The listing builds one solid part. Answer for the finished solid, in the listing's coordinates (mm). Face numbers are marked on the shaded views. Round coordinates to 2 decimals unless told otherwise and drop trailing zeros. Order: outer loops, then holes, each group sorted by start corner. A loop starts at its lowest first (then second) coordinate and runs counter-clockwise, first axis right, second up. Notation, with made-up numbers: M 64,24 L 122,24 A15 ccw 122,28 Z; hole C 48,89 d10. An arc over 180 degrees is marked long. Put each result on its own line as item: value. Start each with the question number.
1. The part is cut by section B-B (x = 0). Count the separate pieces of the cut face and the enclosed holes in it, then the cut area to 3 significant figures.
2. The mould has two halves that part along Y. Classify the marked faces 1 and 2: +Y half, -Y half, draft (parallel to the pull), parting line (faces both ways), or undercut.
3. The part is cut by section A-A (y = 135). Give the vertices of the cut face in (x, z).
4. Consider line 1 (Y direction, x = 0, z = 8.5); line 2 (Y direction, x = -1.5, z = 17.25); line 3 (Y direction, x = 6.5, z = 11.5). Determine where each line is inside the solid, lowest interval first.
5. Each of these flat-tipped pins is pushed along its axis until it touches: pin 1 Ø10 at (y, z) = (74.5, 10.5) entering from -X; pin 2 Ø2.5 at (x, y) = (93, -52) entering from -Z; pin 3 Ø8 at (x, z) = (24, 14.5) entering from -Y; pin 4 Ø16 at (x, y) = (0, 135) entering from -Z. Where does it stop, or does it pass through?
from build123d import *

# Parameters (mm, degrees)
SKETCH1_R           = 152
SKETCH1_R_2         = 86
BOSS_EXTRUDE3_DEPTH = 24
CUT_EXTRUDE6_START  = -7.5
SKETCH5_R           = 152
SKETCH5_R_2         = 112.5
CUT_EXTRUDE6_DEPTH  = 7.5
SKETCH6_R           = 103.5
CUT_EXTRUDE7_DEPTH  = 6
CHAMFER1_SIZE       = 1
SKETCH8_R           = 117
CUT_EXTRUDE8_DEPTH  = 2
SKETCH16_R          = 100
CUT_EXTRUDE9_DEPTH  = 11
CHAMFER3_SIZE       = 1
SKETCH19_R          = 4
CUT_EXTRUDE12_DEPTH = 11
CIRPATTERN1_COUNT   = 6
SKETCH3_R           = 8.75
CUT_EXTRUDE13_DEPTH = 217.296093354
CIRPATTERN2_COUNT   = 8


with BuildPart() as part:
    # Sketch1 → Boss-Extrude3 (new body)
    with BuildSketch(Plane.XY):
        Circle(SKETCH1_R)
        Circle(SKETCH1_R_2, mode=Mode.SUBTRACT)
    extrude(amount=BOSS_EXTRUDE3_DEPTH)

    # Sketch5 → Cut-Extrude6 (cut)
    with BuildSketch(Plane.XY.offset(24).offset(CUT_EXTRUDE6_START)):
        Circle(SKETCH5_R)
        Circle(SKETCH5_R_2, mode=Mode.SUBTRACT)
    extrude(amount=CUT_EXTRUDE6_DEPTH, mode=Mode.SUBTRACT)

    # Sketch6 → Cut-Extrude7 (cut)
    with BuildSketch(Plane.XY.offset(24)):
        Circle(SKETCH6_R)
    extrude(amount=-CUT_EXTRUDE7_DEPTH, mode=Mode.SUBTRACT)

    # Chamfer1
    chamfer1_edges = [part.edges().sort_by_distance(p)[0] for p in [
        (-112.5, 0, 24),
    ]]
    chamfer(chamfer1_edges, length=CHAMFER1_SIZE)

    # Sketch8 → Cut-Extrude8 (cut)
    with BuildSketch(Plane(origin=(0, 0, 0), x_dir=(-1, 0, 0), z_dir=(0, 0, -1))):
        Circle(SKETCH8_R)
    extrude(amount=-CUT_EXTRUDE8_DEPTH, mode=Mode.SUBTRACT)

    # Sketch16 → Cut-Extrude9 (cut)
    with BuildSketch(Plane(origin=(0, 0, 2), x_dir=(-1, 0, 0), z_dir=(0, 0, -1))):
        Circle(SKETCH16_R)
    extrude(amount=-CUT_EXTRUDE9_DEPTH, mode=Mode.SUBTRACT)

    # Chamfer3
    chamfer3_edges = [part.edges().sort_by_distance(p)[0] for p in [
        (100, 0, 2),
    ]]
    chamfer(chamfer3_edges, length=CHAMFER3_SIZE)

    # Sketch19 → Cut-Extrude12 (cut)
    with BuildSketch(Plane(origin=(0, 0, 2), x_dir=(-1, 0, 0), z_dir=(0, 0, -1))):
        with Locations((0, 107.5)):
            Circle(SKETCH19_R)
    cut_extrude12 = extrude(amount=-CUT_EXTRUDE12_DEPTH, mode=Mode.SUBTRACT)

    # CirPattern1: Cut-Extrude12 ×6 about axis
    cirpattern1_axis = Axis((0, 0, 0), (0, 0, 1))
    for i in range(1, CIRPATTERN1_COUNT):
        add(cut_extrude12.rotate(cirpattern1_axis, i * 360 / CIRPATTERN1_COUNT), mode=Mode.SUBTRACT)

    # Sketch3 → Cut-Extrude13 (cut, through all)
    with BuildSketch(Plane(origin=(0, 0, 0), x_dir=(-1, 0, 0), z_dir=(0, 0, -1))):
        with Locations((0, 135)):
            Circle(SKETCH3_R)
    cut_extrude13 = extrude(amount=-CUT_EXTRUDE13_DEPTH, mode=Mode.SUBTRACT)

    # CirPattern2: Cut-Extrude13 ×8 about axis
    cirpattern2_axis = Axis((0, 0, 0), (0, 0, 1))
    for i in range(1, CIRPATTERN2_COUNT):
        add(cut_extrude13.rotate(cirpattern2_axis, i * 360 / CIRPATTERN2_COUNT), mode=Mode.SUBTRACT)


solid = part.part
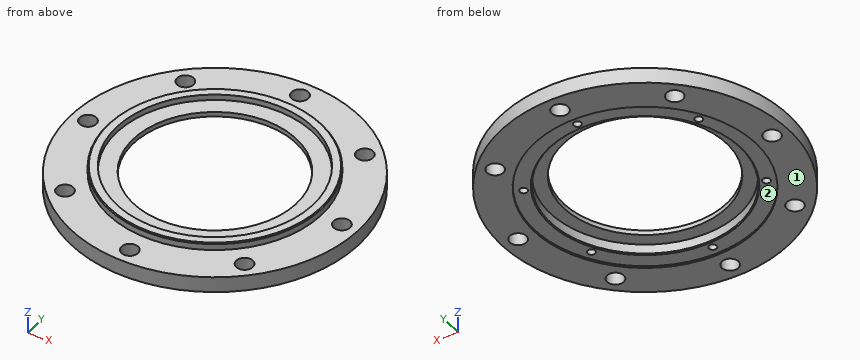
Resolved:
1. separate pieces: 4
1. enclosed holes: 0
1. area: 1,180 mm2
2. face 1: draft
2. face 2: undercut
3. outline: M -69.85,0 L -8.75,0 L -8.75,16.5 L -69.85,16.5 Z; M 8.75,0 L 69.85,0 L 69.85,16.5 L 8.75,16.5 Z
4. line 1: -152 to -143.75, -126.25 to -111.5, -103.5 to -100, 100 to 103.5, 111.5 to 126.25, 143.75 to 152
4. line 2: -112.49 to -85.99, 85.99 to 112.49
4. line 3: -151.86 to -140.86, -129.14 to -99.79, 99.79 to 129.14, 140.86 to 151.86
5. pin 1: x = -135.18
5. pin 2: z = 13
5. pin 3: y = -150.68
5. pin 4: through
